Build history of the part. All positions in model axes, mm. Face numbers are marked on the shaded views. A direction names the side the tool comes from. Give positions to 0.01 mm unless a question says otherwise; leave off trailing zeros. Loops run counter-clockwise (first coordinate to the right, second up) from the corner with the lowest first, then second, coordinate; pieces in that order, holes last. Notation, with made-up numbers: (-16, 43.5) - (23, 43.5) arc R18 ccw to (23, 60.5) - close; hole circle Ø10 at (77, -9). An arc over 180 degrees is marked (long way). Return JSON: item names as keys, results as strings. Group by question number.
1) Slice it at A-A (z = -29.5). List the corners of the cut face in (x, y), and give its area (3 significant figures).
2) Drop flat-ended pins along their axis: pin 1 (1.5 mm diameter, centred on x = -94.5, z = -31, fed in from +Y); pin 2 (5 mm diameter, centred on y = 69.5, z = -9.5, fed in from +X); pin 3 (10 mm diameter, centred on x = -36.5, z = -20.5, fed in from +Y). Give the stop position or say it passes through.
3) Drill centre lines: probe 1 along Z at (x, y) = (-109, 104.5); probe 2 along Y at (x, z) = (-99, -14.5); probe 3 along X at (y, z) = (150.5, -15). Where is each one in solid material? Low to high. Write a range as from..to.
4) Slice it at B-B (y = 10). List the corners of the cut face in (x, z), and give its area (3 significant figures).
5) 3-axis set-ups, long thin cutter, end or side, ignore diameter. For the marked faces 1 and 2: which of +Z, -Z, +X, -X, +Y, -Y reach the whole face in a straight line?
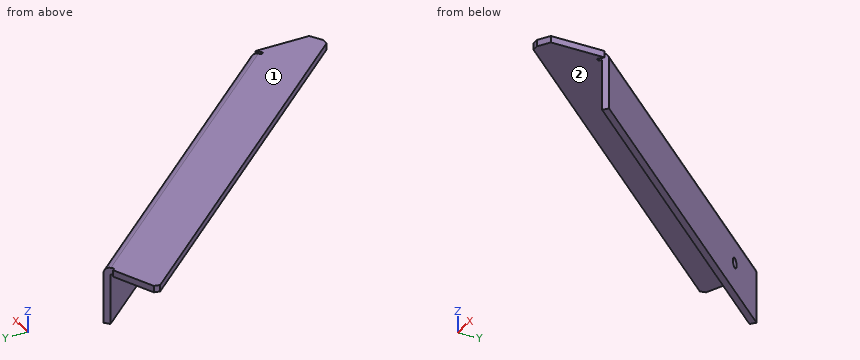
```python
from build123d import *

# Parameters (mm, degrees)
BASE_FLANGE1_DEPTH            = 4
EDGE_FLANGE1_STRIP_W          = 16.4
EDGE_FLANGE1_STRIP_H          = 4
EDGE_FLANGE1_STRIP_CUT_DEPTH  = 236.766242904
EDGE_FLANGE1_RELIEF_W         = 18.4
EDGE_FLANGE1_RELIEF_H         = 2
EDGE_FLANGE1_RELIEF_CUT_DEPTH = 4
EDGE_FLANGE1_DEPTH            = 236.766242904
SKETCH9_R                     = 3
CUT_EXTRUDE1_DEPTH            = 10


# Sheet-metal steps are written as plain solids
with BuildPart() as part:
    # Sketch1 → Base-Flange1 (new body)
    with BuildSketch(Plane.XY):
        Polygon((0, 22.5), (-158.455818563, 198.426141726), (-189.121858967, 184.45082196), (-189.843992647, 180.977630435), (-11.076158097, -17.5), (-7.076158097, -17.5), (0, -12.935441332), align=None)
    extrude(amount=-BASE_FLANGE1_DEPTH)

    # Edge-Flange1 strip (across the edge) → Edge-Flange1 strip cut (cut)
    with BuildSketch(Plane(origin=(-158.455818563, 198.426141726, -4), x_dir=(-0.7430372656499554, -0.6692500443447409, -3.4914813388431334e-15), z_dir=(0.6692500443447409, -0.7430372656499554, 0))):
        with Locations((-4, -2)):
            Rectangle(EDGE_FLANGE1_STRIP_W, EDGE_FLANGE1_STRIP_H)
    extrude(amount=EDGE_FLANGE1_STRIP_CUT_DEPTH, mode=Mode.SUBTRACT)

    # Edge-Flange1 relief (on the sheet) → Edge-Flange1 relief cut (cut)
    with BuildSketch(Plane(origin=(-161.576575079, 195.615291539, -4), x_dir=(-0.7430372656499554, -0.6692500443447409, -6.982962677686267e-15), z_dir=(0, 0, -1))):
        with Locations((-7.2, 1)):
            Rectangle(EDGE_FLANGE1_RELIEF_W, EDGE_FLANGE1_RELIEF_H)
        with Locations((-7.2, -237.766242904)):
            Rectangle(EDGE_FLANGE1_RELIEF_W, EDGE_FLANGE1_RELIEF_H)
    extrude(amount=-EDGE_FLANGE1_RELIEF_CUT_DEPTH, mode=Mode.SUBTRACT)

    # Edge-Flange1 section (across the edge) → Edge-Flange1 (add)
    with BuildSketch(Plane(origin=(-158.455818563, 198.426141726, -4), x_dir=(-0.7430372656499554, -0.6692500443447409, -3.4914813388431334e-15), z_dir=(0.6692500443447409, -0.7430372656499554, 0))):
        with BuildLine():
            Line((0, 0.2), (0, 31))
            Line((0, 31), (4, 31))
            Line((4, 31), (4, 0.2))
            ThreePointArc((4, 0.2), (4.058578644, 0.058578644), (4.2, 0))
            Line((4.2, 0), (4.2, -4))
            ThreePointArc((4.2, -4), (1.230151519, -2.769848481), (0, 0.2))
        make_face()
    extrude(amount=EDGE_FLANGE1_DEPTH)

    # Sketch9 → Cut-Extrude1 (cut)
    with BuildSketch(Plane(origin=(11.188748767, 10.077651492, 0), x_dir=(0, 0, -1), z_dir=(0.7430372656499554, 0.6692500443447409, -3.560476072298782e-15))):
        with Locations(Location((17.5, 218.484581381, 0), (0, 0, 90))):
            Circle(SKETCH9_R)
    extrude(amount=-CUT_EXTRUDE1_DEPTH, mode=Mode.SUBTRACT)


solid = part.part
```
Results:
{
 "1": {"outline": "(-161.43, 195.75) - (-2.97, 19.82) - (0, 22.5) - (-158.46, 198.43) - close", "area": "947 mm2"},
 "2": {"pin 1": "y = 128.25", "pin 2": "x = -40.08", "pin 3": "y = 68.58"},
 "3": {"probe 1": "-4..0", "probe 2": "126.44..132.42", "probe 3": "-120.67..-115.29"},
 "4": {"outline": "(-35.85, -4) - (0, -4) - (0, 0) - (-35.85, 0) - close", "area": "143 mm2"},
 "5": {"face 1": "+Z, +X, -X, +Y, -Y", "face 2": "-Z, -X, -Y"}
}
